from build123d import *

# Parameters (mm, degrees)
SKETCH1_R           = 6.25
BOSS_EXTRUDE1_DEPTH = 3


with BuildPart() as part:
    # Sketch1 → Boss-Extrude1 (new, symmetric)
    with BuildSketch(Plane(origin=(0, 0, 0), x_dir=(1, 0, 0), z_dir=(0, 1, 0))):
        Polygon((-19, 10), (-16, 10), (-16, -10), (-19, -10), (-19, -12.5), (19, -12.5), (19, 12.5), (-19, 12.5), align=None)
        with Locations(Location((3, 0, 0), (0, 0, 270))):
            Circle(SKETCH1_R, mode=Mode.SUBTRACT)
    extrude(amount=BOSS_EXTRUDE1_DEPTH, both=True)


solid = part.part
Work out the finished part from the listing and answer in its coordinate system (mm). A direction names the side the tool comes from. Give positions to 0.01 mm unless a question says otherwise; leave off trailing zeros. Loops run counter-clockwise (first coordinate to the right, second up) from the corner with the lowest first, then second, coordinate; pieces in that order, holes last. Notation, with made-up numbers: (37, 37) - (62, 37) arc R15 ccw to (62, 55) - close; hole circle Ø6 at (51, 10). An arc over 180 degrees is marked (long way). Answer in a Markdown table with one row per item. Add a question column.
Q1. The part is cut by section B-B (y = 1.65). Determine the outline of the cut face in (x, z).
Q2. A tool of negligible diameter and unlimited length cuts with its end or side. For faces 4 (the flat face through (-16, 0, 0)), 5 (the flat face through (-19, 0, 11)), from which of +Z, -Z, +X, -X, +Y, -Y can it reach the whole face along a straight path? Write none if from no direction.
Q3. Determine the mould class of faces 1 (the flat face through (-19, 0, -11)), 2 (the flat face through (0, 0, 12.5)), 3 (the flat face through (-18, 0, -10)) for opening direction Z: released by +Z, released by -Z, zero draft, split by the parting line, or undercut.
Q4. Consider line 1 along X through (y, z) = (1.8, 0.25) (3 decimals); line 2 along X through (y, z) = (-0.35, 9); line 3 along X through (y, z) = (-1.3, 5.75). Determine where each line is inside the solid, lowest interval first.
Q5. The part is cut by section D-D (z = -7.5). Determine the outline of the cut face in (x, y), and give its area (3 significant figures).
Q6. The part is cut by section A-A (z = 0). Determine the outline of the cut face in (x, y), and give its area (3 significant figures).
Q7. This flat-tipped pin is pushed along its axis until it touches: P1, Ø1.8, axis at y = -1, z = 1.5, coming from the -X side. Where does it stop, or does it pass through?
Q8. The part is cut by section C-C (x = 3). Determine the outline of the cut face in (y, z), and give its area (3 significant figures).
Solution:
| question | item | result |
|---|---|---|
| 1 | outline | (-19, -12.5) - (19, -12.5) - (19, 12.5) - (-19, 12.5) - (-19, 10) - (-16, 10) - (-16, -10) - (-19, -10) - close; hole circle Ø12.5 at (3, 0) |
| 2 | face 4 | -X, +Y, -Y |
| 2 | face 5 | +Z, -Z, -X, +Y, -Y |
| 3 | face 1 | zero draft |
| 3 | face 2 | released by +Z |
| 3 | face 3 | undercut |
| 4 | line 1 | x = -16 to -3.245, 9.245 to 19 |
| 4 | line 2 | x = -16 to 19 |
| 4 | line 3 | x = -16 to 0.55, 5.45 to 19 |
| 5 | outline | (-16, -3) - (19, -3) - (19, 3) - (-16, 3) - close |
| 5 | area | 210 mm² |
| 6 | outline | (-16, -3) - (-3.25, -3) - (-3.25, 3) - (-16, 3) - close; (9.25, -3) - (19, -3) - (19, 3) - (9.25, 3) - close |
| 6 | area | 135 mm² |
| 7 | P1 | stops at x = -16 |
| 8 | outline | (-3, -12.5) - (3, -12.5) - (3, -6.25) - (-3, -6.25) - close; (-3, 6.25) - (3, 6.25) - (3, 12.5) - (-3, 12.5) - close |
| 8 | area | 75.0 mm² |
